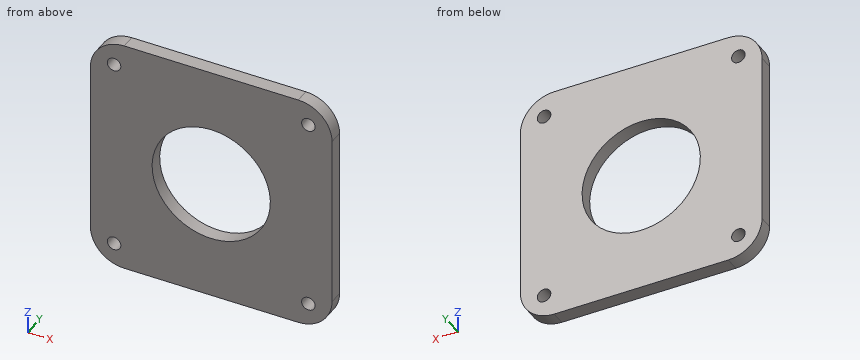
from build123d import *

# Parameters (mm, degrees)
SKETCH1_W           = 71.5
SKETCH1_H           = 71.5
BOSS_EXTRUDE1_DEPTH = 4.2
FILLET1_R           = 10
SKETCH2_R           = 17.5
CUT_EXTRUDE1_DEPTH  = 51.732287549
SKETCH3_R           = 2
CUT_EXTRUDE2_DEPTH  = 51.732287549


with BuildPart() as part:
    # Sketch1 → Boss-Extrude1 (new body)
    with BuildSketch(Plane(origin=(0, 0, 0), x_dir=(1, 0, 0), z_dir=(0, 1, 0))):
        Rectangle(SKETCH1_W, SKETCH1_H)
    extrude(amount=BOSS_EXTRUDE1_DEPTH)

    # Fillet1
    fillet1_edges = [part.edges().sort_by_distance(p)[0] for p in [
        (35.75, 2.1, 35.75),
        (-35.75, 2.1, 35.75),
        (-35.75, 2.1, -35.75),
        (35.75, 2.1, -35.75),
    ]]
    fillet(fillet1_edges, radius=FILLET1_R)

    # Sketch2 → Cut-Extrude1 (cut, through all)
    with BuildSketch(Plane(origin=(0, 4.2, 0), x_dir=(1, 0, 0), z_dir=(0, 1, 0))):
        with Locations(Location((0, 0, 0), (0, 0, 270))):
            Circle(SKETCH2_R)
    extrude(amount=-CUT_EXTRUDE1_DEPTH, mode=Mode.SUBTRACT)

    # Sketch3 → Cut-Extrude2 (cut, through all)
    with BuildSketch(Plane(origin=(0, 4.2, 0), x_dir=(1, 0, 0), z_dir=(0, 1, 0))):
        with Locations(Location((-28.75, 28.75, 0), (0, 0, 270))):
            Circle(SKETCH3_R)
        with Locations(Location((28.75, 28.75, 0), (0, 0, 270))):
            Circle(SKETCH3_R)
        with Locations(Location((-28.75, -28.75, 0), (0, 0, 270))):
            Circle(SKETCH3_R)
        with Locations(Location((28.75, -28.75, 0), (0, 0, 270))):
            Circle(SKETCH3_R)
    extrude(amount=-CUT_EXTRUDE2_DEPTH, mode=Mode.SUBTRACT)


solid = part.part
CAD build for the part. Positions are in the model's coordinates, mm. Coordinates: 2 decimals unless noted, no trailing zeros. Order: outer loops, then holes, each group sorted by start corner. A loop starts at its lowest first (then second) coordinate and runs counter-clockwise, first axis right, second up. Notation, with made-up numbers: (61, -6) -> (76, -6) arc R12 ccw to (76, 7) -> close; hole circle Ø7 at (29.25, 89.5). An arc over 180 degrees is marked (long way). Answer in a Markdown table with one row per item.
1) Band-saw the part on D-D (z = 28.75). List the corners of the cut face in (x, y), and give its area (3 significant figures).
Check values:
| item | result |
|---|---|
| outline | (-35.29, 0) -> (-30.75, 0) -> (-30.75, 4.2) -> (-35.29, 4.2) -> close; (-26.75, 0) -> (26.75, 0) -> (26.75, 4.2) -> (-26.75, 4.2) -> close; (30.75, 0) -> (35.29, 0) -> (35.29, 4.2) -> (30.75, 4.2) -> close |
| area | 263 mm2 |
2) Drill centre lines: line 1 (X direction, y = 2.6, z = 0); line 2 (X direction, y = 1.55, z = -28.5); line 3 (X direction, y = 1.7, z = -28.75). Where is each one in solid material? Low to high.
Check values:
| item | result |
|---|---|
| line 1 | -35.75 to -17.5, 17.5 to 35.75 |
| line 2 | -35.36 to -30.73, -26.77 to 26.77, 30.73 to 35.36 |
| line 3 | -35.29 to -30.75, -26.75 to 26.75, 30.75 to 35.29 |
3) Band-saw the part on C-C (x = -28.75). List the corners of the cut face in (y, z).
Check values:
| item | result |
|---|---|
| outline | (0, -35.29) -> (4.2, -35.29) -> (4.2, -30.75) -> (0, -30.75) -> close; (0, -26.75) -> (4.2, -26.75) -> (4.2, 26.75) -> (0, 26.75) -> close; (0, 30.75) -> (4.2, 30.75) -> (4.2, 35.29) -> (0, 35.29) -> close |
4) Flat gauge pin, fed straight in: P1, Ø1, axis at y = 1, z = 27, coming from the -X side. Where does the tip first touch, or does it go through?
Check values:
| item | result |
|---|---|
| P1 | x = -35.72 |
5) Band-saw the part on A-A (z = 14). List the corners of the cut face in (x, y).
Check values:
| item | result |
|---|---|
| outline | (-35.75, 0) -> (-10.5, 0) -> (-10.5, 4.2) -> (-35.75, 4.2) -> close; (10.5, 0) -> (35.75, 0) -> (35.75, 4.2) -> (10.5, 4.2) -> close |
6) Band-saw the part on B-B (y = 2.5). List the corners of the cut face in (x, z), and give its area (3 significant figures).
Check values:
| item | result |
|---|---|
| outline | (-35.75, -25.75) arc R10 ccw to (-25.75, -35.75) -> (25.75, -35.75) arc R10 ccw to (35.75, -25.75) -> (35.75, 25.75) arc R10 ccw to (25.75, 35.75) -> (-25.75, 35.75) arc R10 ccw to (-35.75, 25.75) -> close; hole circle Ø4 at (-28.75, -28.75); hole circle Ø4 at (-28.75, 28.75); hole circle Ø35 at (0, 0); hole circle Ø4 at (28.75, -28.75); hole circle Ø4 at (28.75, 28.75) |
| area | 4,010 mm2 |
